Geometry check sheet. Reference: the model listing, model coordinates, mm. A direction names the side the tool comes from. Round coordinates to 2 decimals unless told otherwise and drop trailing zeros. Order: outer loops, then holes, each group sorted by start corner. A loop starts at its lowest first (then second) coordinate and runs counter-clockwise, first axis right, second up. Notation, with made-up numbers: (80, 78) - (139, 78) arc R14 cw to (139, 104) - close; hole circle Ø7 at (81, 5). An arc over 180 degrees is marked (long way). Answer as CSV lines item,"result". Start each with the question number.
```python
from build123d import *

# Parameters (mm, degrees)
MODEL_W                 = 10
MODEL_H                 = 3
MODEL_W_2               = 3
MODEL_H_2               = 10
MODEL_R                 = 1.5
SALIENTE_EXTRUIR1_DEPTH = 3


with BuildPart() as part:
    # Model → Saliente-Extruir1 (new body)
    with BuildSketch(Plane.XY):
        with BuildLine():
            Line((-10.274239299, -47.526259687), (-5.274229553, -47.526259687))
            ThreePointArc((-5.274229553, -47.526259687), (1.796838258, -50.455191875), (4.725770447, -57.526259687))
            Line((4.725770447, -57.526259687), (4.725770447, -57.532159687))
            ThreePointArc((4.725770447, -57.532159687), (7.654702635, -64.603227499), (14.725770447, -67.532159687))
            Line((14.725770447, -67.532159687), (74.725770447, -67.532159687))
            ThreePointArc((74.725770447, -67.532159687), (81.796838258, -64.603227499), (84.725770447, -57.532159687))
            Line((84.725770447, -57.532159687), (84.725770447, -57.526259687))
            ThreePointArc((84.725770447, -57.526259687), (87.654702635, -50.455191875), (94.725770447, -47.526259687))
            Line((94.725770447, -47.526259687), (99.732474793, -47.526259687))
            ThreePointArc((99.732474793, -47.526259687), (106.803542605, -44.597327499), (109.732474793, -37.526259687))
            Line((109.732474793, -37.526259687), (109.732474793, 64.073740313))
            ThreePointArc((109.732474793, 64.073740313), (106.803542605, 71.144808125), (99.732474793, 74.073740313))
            Line((99.732474793, 74.073740313), (49.729117747, 74.073740313))
            ThreePointArc((49.729117747, 74.073740313), (47.772685887, 82.360468062), (50.374223429, 90.467840313))
            ThreePointArc((50.374223429, 90.467840313), (42.906482031, 83.66371575), (39.729117747, 74.073740313))
            Line((39.729117747, 74.073740313), (-10.274239299, 74.073740313))
            ThreePointArc((-10.274239299, 74.073740313), (-17.345307111, 71.144808125), (-20.274239299, 64.073740313))
            Line((-20.274239299, 64.073740313), (-20.274239299, -37.526259687))
            ThreePointArc((-20.274239299, -37.526259687), (-17.345307111, -44.597327499), (-10.274239299, -47.526259687))
        make_face()
        Polygon((-4.710690354, -40.763410741), (-13.511389214, -31.962709682), (3.012309414, -15.439007345), (11.813010679, -24.239709709), align=None, mode=Mode.SUBTRACT)
        with Locations((30.725760701, -60.959219621)):
            Rectangle(MODEL_W, MODEL_H, mode=Mode.SUBTRACT)
        with Locations((-13.08093725, -9.772535148)):
            Rectangle(MODEL_W_2, MODEL_H_2, mode=Mode.SUBTRACT)
        with Locations((14.984988274, -12.305130612)):
            Circle(MODEL_R, mode=Mode.SUBTRACT)
        Polygon((63.725774778, -62.459219621), (53.725780192, -62.459219621), (53.725780192, -59.459219621), (63.725774778, -59.448813721), align=None, mode=Mode.SUBTRACT)
        Polygon((102.969574793, -31.962759687), (94.16892376, -40.763410719), (77.645224816, -24.239709664), (86.445874793, -15.439059687), align=None, mode=Mode.SUBTRACT)
        with Locations((74.511280689, -12.267097017)):
            Circle(MODEL_R, mode=Mode.SUBTRACT)
        with Locations((99.91359519, -9.772535148)):
            Rectangle(MODEL_W_2, MODEL_H_2, mode=Mode.SUBTRACT)
        with Locations((-13.08093725, 36.320015775)):
            Rectangle(MODEL_W_2, MODEL_H_2, mode=Mode.SUBTRACT)
        with Locations((14.984988274, 38.81446274)):
            Circle(MODEL_R, mode=Mode.SUBTRACT)
        Polygon((-4.710739299, 67.310840313), (11.812961756, 50.787139259), (3.012310656, 41.986490358), (-13.511389299, 58.510190313), align=None, mode=Mode.SUBTRACT)
        with Locations((74.511280689, 38.81446274)):
            Circle(MODEL_R, mode=Mode.SUBTRACT)
        with Locations((99.91359519, 36.320015775)):
            Rectangle(MODEL_W_2, MODEL_H_2, mode=Mode.SUBTRACT)
        Polygon((103.007708555, 58.472006804), (86.39069839, 41.854996145), (77.551864592, 50.693831877), (94.168873658, 67.310841438), align=None, mode=Mode.SUBTRACT)
    extrude(amount=SALIENTE_EXTRUIR1_DEPTH)


solid = part.part
```
1. Section check D-D on y = 77. Record the boundary of the cut face in (x, z).
2. Section check C-C on z = 2.25. Count the separate pieces of the cut face and the enclosed holes in it, plus the area to 3 significant figures.
3. Access from +Z, -Z, +X, -X, +Y, -Y to the whole of each face (thin tool, end or side, straight path). Record for faces 4 (the face through (94.592, -23.585, 1.479)), 5 (the face through (44, 13, 0)).
4. Section check B-B on x = 9.5. Record the boundary of the cut face in (y, z), plus the area to 3 significant figures.
5. Draft check along Y on faces 1 (the face through (-5.37, -23.82, 1.48)), 2 (the face through (81.7, -64.7, 1.5)), 3 (the face through (-17.27, 71.22, 1.48)). Enter one of: released by +Y, released by -Y, zero draft, split by the parting line, or undercut.
6. Thickness scan on probe 1 along X at (y, z) = (-14, 2.45); probe 2 along Y at (x, z) = (6.5, 0.45); probe 3 along X at (y, z) = (49.5, 1.7). Record the ranges inside material, lowest first.
7. Section check A-A on y = 34.5. Record the boundary of the cut face in (x, z).
8. Go/stop test with flat-tipped pins: pin 1 Ø0.9 at (x, z) = (-9, 1) entering from -Y; pin 2 Ø0.9 at (y, z) = (-60.5, 1.5) entering from +X; pin 3 Ø1.5 at (x, z) = (99, 1) entering from +Y. Record where each tip stops, or that it passes through.
Numbers:
1,outline,"(40.14, 0) - (48.48, 0) - (48.48, 3) - (40.14, 3) - close"
2,separate pieces,"1"
2,enclosed holes,"14"
2,area,"16,000 mm2"
3,face 4,"+Z, -Z"
3,face 5,"-Z, +X, -X, +Y, -Y"
4,outline,"(-66.06, 0) - (-26.55, 0) - (-26.55, 3) - (-66.06, 3) - close; (-21.93, 0) - (48.47, 0) - (48.47, 3) - (-21.93, 3) - close; (53.1, 0) - (74.07, 0) - (74.07, 3) - (53.1, 3) - close"
4,area,"393 mm2"
5,face 1,"undercut"
5,face 2,"released by -Y"
5,face 3,"released by +Y"
6,probe 1,"x = -20.27 to -14.58, -11.58 to 98.41, 101.41 to 109.73"
6,probe 2,"y = -63.22 to -29.55, -18.93 to 45.47, 56.1 to 74.07"
6,probe 3,"x = -20.27 to -4.5, 10.53 to 78.75, 94.04 to 109.73"
7,outline,"(-20.27, 0) - (-14.58, 0) - (-14.58, 3) - (-20.27, 3) - close; (-11.58, 0) - (98.41, 0) - (98.41, 3) - (-11.58, 3) - close; (101.41, 0) - (109.73, 0) - (109.73, 3) - (101.41, 3) - close"
8,pin 1,"stops at y = -47.53"
8,pin 2,"stops at x = 84.4"
8,pin 3,"stops at y = 74.07"
